```python
from build123d import *

# Parameters (mm, degrees)
PAD_DEPTH       = 16
SKETCH002_R     = 2.15
POCKET001_DEPTH = 8
SKETCH003_R     = 2.15
POCKET002_DEPTH = 8
PAD001_DEPTH    = 62
SKETCH005_W     = 723.80365
SKETCH005_H     = 658.353257
POCKET003_DEPTH = 30
CHAMFER_SIZE    = 1
SKETCH001_R     = 2.15
SKETCH001_W     = 2.6
SKETCH001_H     = 6
POCKET_DEPTH    = 62.001
SKETCH006_W     = 116
SKETCH006_H     = 16
PAD002_DEPTH    = 2


with BuildPart() as part:
    # Sketch → Pad (new body)
    with BuildSketch(Plane.XY):
        Polygon((0, 0), (0, 43), (27.6, 43), (27.6, 28), (47.6, 28), (47.6, 43), (76.6, 43), (76.6, 31), (152.2, 31), (152.2, 0), align=None)
    extrude(amount=PAD_DEPTH)

    # Sketch002 → Pocket001 (cut)
    with BuildSketch(Plane.YZ):
        with Locations((12, 8)):
            Circle(SKETCH002_R)
    extrude(amount=POCKET001_DEPTH, mode=Mode.SUBTRACT)

    # Sketch003 (on DatumPlane) → Pocket002 (cut)
    with BuildSketch(Plane.YZ.offset(152.2)):
        with Locations((12, 8)):
            Circle(SKETCH003_R)
    extrude(amount=-POCKET002_DEPTH, mode=Mode.SUBTRACT)

    # Sketch004 → Pad001 (join)
    with BuildSketch(Plane.XZ):
        Polygon((128, 0), (152.2, 0), (152.2, -5), (133, -5), (133, -60), (139.919662, -60), (139.919662, -69), (152.2, -69), (152.2, -85), (128, -85), (128, -68), (134.5, -68), (134.5, -65), (128, -65), align=None)
        Polygon((0, 0), (12, 0), (12, -65), (5.5, -65), (5.5, -68), (12, -68), (12, -85), (0, -85), (0, -65), align=None)
    extrude(amount=-PAD001_DEPTH)

    # Sketch005 → Pocket003 (cut)
    with BuildSketch(Plane.XY):
        with Locations((105.388489, 130.509316)):
            Rectangle(SKETCH005_W, SKETCH005_H)
        Polygon((0, 0), (0, 43), (76.6, 43), (76.6, 31), (152.2, 31), (152.2, 0), align=None, mode=Mode.SUBTRACT)
    extrude(amount=-POCKET003_DEPTH, mode=Mode.SUBTRACT)

    # Chamfer
    chamfer_edges = [part.edges().sort_by_distance(p)[0] for p in [
        (133, 46.5, -30),
        (133, 15.5, -5),
        (128, 31, -15),
        (128, 62, -47.5),
        (27.6, 35.5, 0),
        (0, 9.85, 8),
    ]]
    chamfer(chamfer_edges, length=CHAMFER_SIZE)

    # Sketch001 → Pocket (cut, through all)
    with BuildSketch(Plane.XZ):
        with Locations((12, 8)):
            Circle(SKETCH001_R)
        with Locations((89.6, 8)):
            Circle(SKETCH001_R)
        with Locations((140.2, 8)):
            Circle(SKETCH001_R)
        with Locations((57.6, 8)):
            Circle(SKETCH001_R)
        with Locations((140.2, -77)):
            Circle(SKETCH001_R)
        with Locations((21.3, 13)):
            Rectangle(SKETCH001_W, SKETCH001_H)
        with Locations((130.9, 13)):
            Rectangle(SKETCH001_W, SKETCH001_H)
    extrude(amount=-POCKET_DEPTH, mode=Mode.SUBTRACT)

    # Sketch006 → Pad002 (join)
    with BuildSketch(Plane.XZ):
        with Locations((70, -77)):
            Rectangle(SKETCH006_W, SKETCH006_H)
    extrude(amount=-PAD002_DEPTH)


solid = part.part
```
Source: CAD feature listing. Evaluate the final solid. Frame: model axes, mm. A direction names the side the tool comes from. Round coordinates to 2 decimals unless told otherwise and drop trailing zeros. Loops run counter-clockwise (first coordinate to the right, second up) from the corner with the lowest first, then second, coordinate; pieces in that order, holes last. Notation, with made-up numbers: M 20,49 L 71,49 A16 cw 71,77 Z; hole C 14,-39.75 d5. An arc over 180 degrees is marked long. Use a Markdown table: item, result. Add a question column.
1. Section query A-A on x = 105.5. Return the cut outline in (y, z), then the cut area to 3 significant figures.
2. Mould query, pull axis Y, two halves, no side actions, for faces 1 (the flat face through (133, 24, -39)), 2 (the cylindrical face through (4.45, 13.16, 9.81)), 3 (the flat face through (69, 2, -77)). Classes: pulls with the +Y half, pulls with the -Y half, needs draft (parallel to the pull), parting line crosses it, or undercut.
3. Reachability of faces 4 (the flat face through (6, 53, -30)), 5 (the flat face through (122, 31, 3)), 6 (the flat face through (131, 31, -68)) from +Z, -Z, +X, -X, +Y, -Y: full face, straight path, thin tool, end or side. Return the list, or none.
4. Line query: line 1 (Z direction, x = 130, y = 7); line 2 (X direction, y = 32, z = -40); line 3 (Z direction, x = 21.5, y = 34.5). Output: solid intervals per line, ascending.
5. Section query C-C on z = -63. Return the cut outline in (x, y).
6. Section query D-D on x = 69.5. Return the cut outline in (y, z).
7. Section query B-B on y = 52.5. Return the cut outline in (x, z), then the cut area to 3 significant figures.
8. Contact query for flat-ended pins moving along their axis: P1, Ø7, axis at x = 140.2, z = 8, coming from the +Y side; P2, Ø1.3, axis at y = 12.5, z = 9, coming from the +X side; P3, Ø12, axis at x = 75, y = 33.5, coming from the -Z side; P4, Ø10, axis at x = 131, z = -22, coming from the -Y side. Output: stop coordinate, or through.
Reported:
| question | item | result |
|---|---|---|
| 1 | outline | M 0,-85 L 2,-85 L 2,-69 L 0,-69 Z; M 0,0 L 31,0 L 31,16 L 0,16 Z |
| 1 | area | 528 mm² |
| 2 | face 1 | needs draft |
| 2 | face 2 | undercut |
| 2 | face 3 | pulls with the +Y half |
| 3 | face 4 | +Z, +X, -X, +Y |
| 3 | face 5 | +Z, +X, +Y |
| 3 | face 6 | +Y, -Y |
| 4 | line 1 | z = -85 to -68, -65 to 10 |
| 4 | line 2 | x = 0 to 12, 128 to 133 |
| 4 | line 3 | z = 0 to 10 |
| 5 | outline | M 0,0 L 12,0 L 12,62 L 0,62 Z; M 128,0 L 139.92,0 L 139.92,62 L 129,62 L 128,61 Z |
| 6 | outline | M 0,-85 L 2,-85 L 2,-69 L 0,-69 Z; M 0,0 L 43,0 L 43,16 L 0,16 Z |
| 7 | outline | M 0,-85 L 12,-85 L 12,-68 L 5.5,-68 L 5.5,-65 L 12,-65 L 12,-30 L 0,-30 Z; M 128,-85 L 152.2,-85 L 152.2,-69 L 139.92,-69 L 139.92,-60 L 133,-60 L 133,-31 L 132,-30 L 128,-30 L 128,-65 L 134.5,-65 L 134.5,-68 L 128,-68 Z; hole C 140.2,-77 d4.3 |
| 7 | area | 1,250 mm² |
| 8 | P1 | stops at y = 31 |
| 8 | P2 | stops at x = 144.2 |
| 8 | P3 | stops at z = 0 |
| 8 | P4 | stops at y = 0 |
